Verification items for the finished model (mm, model axes). Face numbers are marked on the shaded views. A direction names the side the tool comes from. Coordinates: 2 decimals unless noted, no trailing zeros. Order: outer loops, then holes, each group sorted by start corner. A loop starts at its lowest first (then second) coordinate and runs counter-clockwise, first axis right, second up. Notation, with made-up numbers: M 86,23 L 141,23 A13 cw 141,41 Z; hole C 27.25,-8 d5. An arc over 180 degrees is marked long. Return JSON: item names as keys, results as strings. Group by question number.
Q1. Section check D-D, the plane x = -9. Enter the section's corners in (y, z), then the cut area to 3 significant figures.
Q2. Section check C-C, the plane z = 24.7. Enter the section's corners in (x, y), then the cut area to 3 significant figures.
Q3. Mould release check, pull along Y, two halves, no side actions. Record for the marked faces 1, 2 and 3: pulls with the +Y half, pulls with the -Y half, needs draft (parallel to the pull), parting line crosses it, or undercut.
Q4. Access from +Z, -Z, +X, -X, +Y, -Y to the whole of each face (thin tool, end or side, straight path). Record for the marked faces 4, 5 and 6.
Q5. Thickness scan on probe 1 along X at (y, z) = (-9.3, 24.7); probe 2 along X at (y, z) = (-9.65, -24.7); probe 3 along Y at (x, z) = (6.5, 12). Record the ranges inside material, lowest first.
Q6. Go/stop test with flat-tipped pins: pin 1 Ø3.5 at (x, z) = (2, -23.5) entering from -Y; pin 2 Ø4 at (x, z) = (-6, -24.7) entering from -Y; pin 3 Ø7.5 at (x, z) = (-3.5, -24.5) entering from +Y; pin 4 Ø6 at (x, y) = (3, 10.5) entering from -Z. Record where each tip stops, or that it passes through.
Q7. Section check B-B, the plane z = -1.5. Enter the section's corners in (x, y).
Q8. Section check A-A, the plane x = 4.5. Enter the section's corners in (y, z), then the cut area to 3 significant figures.
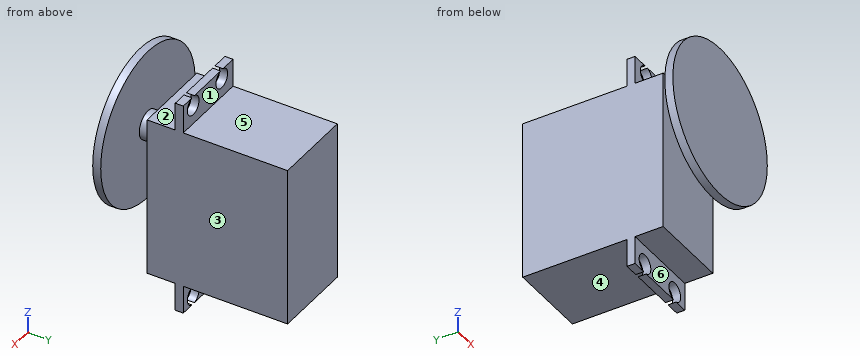
from build123d import *

# Parameters (mm, degrees)
F0_W     = 20
F0_H     = 40
F1_DEPTH = 17.5
F2_W     = 20
F2_H     = 2
F3_DEPTH = 27
F4_R     = 3.5
F5_DEPTH = 8
F6_R     = 19
F7_DEPTH = 2
F8_R     = 2.35
F9_DEPTH = 25.4


with BuildPart() as f1:
    # F0 (on Front) → F1 (new body, symmetric)
    with BuildSketch(Plane.XZ):
        Rectangle(F0_W, F0_H)
    extrude(amount=F1_DEPTH, both=True)

    # F2 (on Top) → F3 (join, symmetric)
    with BuildSketch(Plane.XY):
        with Locations((0, -9.5)):
            Rectangle(F2_W, F2_H)
    extrude(amount=F3_DEPTH, both=True)

    # F4 (on face) → F5 (join)
    with BuildSketch(Plane.XZ.offset(17.5)):
        with Locations((0, 10.5)):
            Circle(F4_R)
    extrude(amount=F5_DEPTH)

    # F6 (on face) → F7 (join)
    with BuildSketch(Plane.XZ.offset(25.5)):
        with Locations((0, 10.5)):
            Circle(F6_R)
    extrude(amount=-F7_DEPTH)

    # F8 (on face) → F9 (cut)
    with BuildSketch(Plane.XZ.offset(10.5)):
        with Locations((-6, -24.7)):
            Circle(F8_R)
        with Locations((6, -24.7)):
            Circle(F8_R)
        with Locations((-5.5, 24.7)):
            Circle(F8_R)
        with Locations((6, 24.7)):
            Circle(F8_R)
    extrude(amount=-F9_DEPTH, mode=Mode.SUBTRACT)


solid = f1.part
Numbers:
{
 "1": {"outline": "M -25.5,-6.23 L -23.5,-6.23 L -23.5,27.23 L -25.5,27.23 Z; M -17.5,-20 L -10.5,-20 L -10.5,-27 L -8.5,-27 L -8.5,-20 L 17.5,-20 L 17.5,20 L -8.5,20 L -8.5,27 L -10.5,27 L -10.5,20 L -17.5,20 Z", "area": "1,490 mm2"},
 "2": {"outline": "M -12.62,-25.5 L 12.62,-25.5 L 12.62,-23.5 L -12.62,-23.5 Z; M -10,-10.5 L -7.85,-10.5 L -7.85,-8.5 L -10,-8.5 Z; M -3.15,-10.5 L 3.65,-10.5 L 3.65,-8.5 L -3.15,-8.5 Z; M 8.35,-10.5 L 10,-10.5 L 10,-8.5 L 8.35,-8.5 Z", "area": "71.7 mm2"},
 "3": {"face 1": "pulls with the +Y half", "face 2": "undercut", "face 3": "needs draft"},
 "4": {"face 4": "-Z, +X, -X, +Y", "face 5": "+Z, +X, -X, +Y", "face 6": "-Z, +X, -X, -Y"},
 "5": {"probe 1": "x = -10 to -7.85, -3.15 to 3.65, 8.35 to 10", "probe 2": "x = -10 to -8.35, -3.65 to 3.65, 8.35 to 10", "probe 3": "y = -25.5 to -23.5, -17.5 to 17.5"},
 "6": {"pin 1": "stops at y = -10.5", "pin 2": "passes through", "pin 3": "stops at y = -8.5", "pin 4": "stops at z = -20"},
 "7": {"outline": "M -14.73,-25.5 L 14.73,-25.5 L 14.73,-23.5 L -14.73,-23.5 Z; M -10,-17.5 L 10,-17.5 L 10,17.5 L -10,17.5 Z"},
 "8": {"outline": "M -25.5,-7.96 L -23.5,-7.96 L -23.5,28.96 L -25.5,28.96 Z; M -17.5,-20 L -10.5,-20 L -10.5,-22.89 L -8.5,-22.89 L -8.5,-20 L 17.5,-20 L 17.5,20 L -8.5,20 L -8.5,22.89 L -10.5,22.89 L -10.5,20 L -17.5,20 Z; M -10.5,-27 L -8.5,-27 L -8.5,-26.51 L -10.5,-26.51 Z; M -10.5,26.51 L -8.5,26.51 L -8.5,27 L -10.5,27 Z", "area": "1,490 mm2"}
}
